Source: CAD feature listing. Evaluate the final solid. Frame: model axes, mm. A direction names the side the tool comes from. Coordinates: 2 decimals unless noted, no trailing zeros. Write each loop counter-clockwise with the first axis right and the second up, starting at its lowest first coordinate (ties: lowest second). Pieces come first, ordered by that corner, then holes. Notation, with made-up numbers: M 0,36 L 21,36 A16 cw 21,66 Z; hole C 16,88.5 d6. An arc over 180 degrees is marked long. One line per item, written item: value. Start each with the question number.
Item 1: Ray query, L1, parallel to Y at x = 3.25, z = -3; L2, parallel to Y at x = 2.5, z = -6.5; L3, parallel to Z at x = -0.25, y = 7.25. Return the intervals inside material, ascending. Write a range as from..to.
Item 2: Cut plane D-D, the plane y = 3.25. Output: boundary loops of the cut face in (x, z).
Item 3: Set-up query: faces 4 (the flat face through (0, 9.7, -8)), 5 (the flat face through (0, 4, -7.4)), 6 (the flat face through (-2.8, 4, -8)), 7 (the cylindrical face through (-6.834, 6.872, -1.517)). Return all of +Z, -Z, +X, -X, +Y, -Y with unobstructed straight access to the full face (end or side cutting, diameter ignored); none if empty.
Item 4: Cut plane B-B, the plane z = -1.5. Output: boundary loops of the cut face in (x, y).
Item 5: Pin query (flat end, axial travel): P1, Ø2.5, axis at x = -1, z = -8, coming from the +Y side; P2, Ø3.5, axis at x = -0.5, y = 3.5, coming from the +Z side; P3, Ø4, axis at y = 6, z = -2.5, coming from the -X side. Return the tip coordinate at first contact, or that it passes through.
Item 6: Cut plane A-A, the plane y = 6.5. Output: boundary loops of the cut face in (x, z).
Item 7: Mould query, pull axis Z, two halves, no side actions, for faces 1 (the cylindrical face through (0.894, 0.76, 10.767)), 2 (the flat face through (2.695, 8, -8)), 3 (the cylindrical face through (9.7, 0.74, 6.18)). Classes: released by +Z, released by -Z, zero draft, split by the parting line, or undercut.
Item 8: Cut plane C-C, the plane x = 0. Output: boundary loops of the cut face in (y, z), then the cut area to 3 significant figures.
```python
from build123d import *

# Parameters (mm, degrees)
ESBO_O1_R                = 11.5
RESSALTO_EXTRUS_O1_DEPTH = 1.5
ESBO_O2_W                = 5.6
ESBO_O2_H                = 2.2
RESSALTO_EXTRUS_O2_DEPTH = 4.5
RESSALTO_EXTRUS_O3_DEPTH = 3.7
ESBO_O4_R                = 1
RESSALTO_EXTRUS_O4_DEPTH = 3.4
ESBO_O5_R                = 7
RESSALTO_EXTRUS_O5_DEPTH = 4
ESBO_O6_R                = 5.830002148
RESSALTO_EXTRUS_O6_DEPTH = 0.5
ESBO_O7_R                = 1
RESSALTO_EXTRUS_O7_DEPTH = 0.5
ESBO_O8_R                = 0.5
CORTE_EXTRUS_O1_DEPTH    = 19.304644219


with BuildPart() as part:
    # Esboço1 → Ressalto-extrusão1 (new body)
    with BuildSketch(Plane(origin=(0, 0, 0), x_dir=(1, 0, 0), z_dir=(0, 1, 0))):
        with Locations(Location((0, 0, 0), (0, 0, 270))):
            Circle(ESBO_O1_R)
    extrude(amount=RESSALTO_EXTRUS_O1_DEPTH)

    # Esboço2 → Ressalto-extrusão2 (add)
    with BuildSketch(Plane(origin=(0, 1.5, 0), x_dir=(1, 0, 0), z_dir=(0, 1, 0))):
        with Locations((0, 8.5)):
            Rectangle(ESBO_O2_W, ESBO_O2_H)
    extrude(amount=RESSALTO_EXTRUS_O2_DEPTH)

    # Esboço3 → Ressalto-extrusão3 (add)
    with BuildSketch(Plane(origin=(0, 6, 0), x_dir=(1, 0, 0), z_dir=(0, 1, 0))):
        with BuildLine():
            Line((-2.695146994, 9.271525864), (2.695146994, 9.271525864))
            Line((2.695146994, 9.271525864), (2.695146994, 7.7))
            ThreePointArc((2.695146994, 7.7), (2.63656835, 7.558578644), (2.495146994, 7.5))
            Line((2.495146994, 7.5), (-2.495146994, 7.5))
            ThreePointArc((-2.495146994, 7.5), (-2.63656835, 7.558578644), (-2.695146994, 7.7))
            Line((-2.695146994, 7.7), (-2.695146994, 9.271525864))
        make_face()
    extrude(amount=RESSALTO_EXTRUS_O3_DEPTH)

    # Esboço4 → Ressalto-extrusão4 (add)
    with BuildSketch(Plane(origin=(0, 1.5, 0), x_dir=(1, 0, 0), z_dir=(0, 1, 0))):
        with Locations(Location((0, 0, 0), (0, 0, 270))):
            Circle(ESBO_O4_R)
    extrude(amount=RESSALTO_EXTRUS_O4_DEPTH)

    # Esboço5 → Ressalto-extrusão5 (add)
    with BuildSketch(Plane(origin=(0, 4.9, 0), x_dir=(1, 0, 0), z_dir=(0, 1, 0))):
        with Locations(Location((0, 0, 0), (0, 0, 270))):
            Circle(ESBO_O5_R)
    extrude(amount=RESSALTO_EXTRUS_O5_DEPTH)

    # Esboço6 → Ressalto-extrusão6 (add)
    with BuildSketch(Plane(origin=(0, 8.9, 0), x_dir=(1, 0, 0), z_dir=(0, 1, 0))):
        with Locations(Location((0, 0, 0), (0, 0, 270))):
            Circle(ESBO_O6_R)
    extrude(amount=RESSALTO_EXTRUS_O6_DEPTH)

    # Esboço7 → Ressalto-extrusão7 (add)
    with BuildSketch(Plane(origin=(0, 9.4, 0), x_dir=(1, 0, 0), z_dir=(0, 1, 0))):
        with Locations(Location((0, 0, 0), (0, 0, 270))):
            Circle(ESBO_O7_R)
    extrude(amount=RESSALTO_EXTRUS_O7_DEPTH)

    # Esboço8 → Corte-extrusão1 (cut, through all)
    with BuildSketch(Plane(origin=(0, 1.5, 0), x_dir=(1, 0, 0), z_dir=(0, 1, 0))):
        with Locations(Location((5.194212024, -8.970404078, 0), (0, 0, 270))):
            Circle(ESBO_O8_R)
        with Locations(Location((3.210199576, -9.853743332, 0), (0, 0, 270))):
            Circle(ESBO_O8_R)
        with Locations(Location((1.085886001, -10.305280121, 0), (0, 0, 270))):
            Circle(ESBO_O8_R)
        with Locations(Location((-1.085886001, -10.305280121, 0), (0, 0, 270))):
            Circle(ESBO_O8_R)
        with Locations(Location((-3.210199576, -9.853743332, 0), (0, 0, 270))):
            Circle(ESBO_O8_R)
        with Locations(Location((-5.194212024, -8.970404078, 0), (0, 0, 270))):
            Circle(ESBO_O8_R)
    extrude(amount=-CORTE_EXTRUS_O1_DEPTH, mode=Mode.SUBTRACT)


solid = part.part
```
From the geometry:
1. L1: y = 0..1.5, 4.9..9.4
1. L2: y = 0..1.5, 4.9..8.9
1. L3: z = -9.27..-7.5, -7..7
2. outline: M -2.8,-9.6 L 2.8,-9.6 L 2.8,-7.4 L -2.8,-7.4 Z; C 0,0 d2
3. face 4: -Z, +X, -X, +Y
3. face 5: +X, -X, +Y
3. face 6: -Z, -X, +Y
3. face 7: +Y
4. outline: M -11.4,0 L 11.4,0 L 11.4,1.5 L -11.4,1.5 Z; M -6.84,4.9 L 6.84,4.9 L 6.84,8.9 L 5.63,8.9 L 5.63,9.4 L -5.63,9.4 L -5.63,8.9 L -6.84,8.9 Z
5. P1: stops at y = 9.7
5. P2: stops at z = 7
5. P3: stops at x = -6.98
6. outline: C 0,0 d14; M -2.7,-9.27 L 2.7,-9.27 L 2.7,-7.7 A0.2 ccw 2.5,-7.5 L -2.5,-7.5 A0.2 ccw -2.7,-7.7 Z
7. face 1: undercut
7. face 2: zero draft
7. face 3: split by the parting line
8. outline: M 0,-11.5 L 1.5,-11.5 L 1.5,-9.6 L 6,-9.6 L 6,-9.27 L 9.7,-9.27 L 9.7,-7.5 L 6,-7.5 L 6,-7.4 L 1.5,-7.4 L 1.5,-1 L 4.9,-1 L 4.9,-7 L 8.9,-7 L 8.9,-5.83 L 9.4,-5.83 L 9.4,-1 L 9.9,-1 L 9.9,1 L 9.4,1 L 9.4,5.83 L 8.9,5.83 L 8.9,7 L 4.9,7 L 4.9,1 L 1.5,1 L 1.5,11.5 L 0,11.5 Z
8. area: 121 mm²
